Can you work these out from the model? Positions are in its coordinate system, mm. Face numbers are marked on the shaded views. A direction names the side the tool comes from. Coordinates: 2 decimals unless noted, no trailing zeros.
```python
from build123d import *

# Parameters (mm, degrees)
SKETCH1_R                    = 9.5
BOSS_EXTRUDE1_DEPTH          = 10
CHAMFER1_SIZE                = 0.75
CIRPATTERN1_COUNT            = 12
CHAMFER1_OF_CIRPATTERN1_SIZE = 0.75
SKETCH2_R                    = 7
SKETCH2_R_2                  = 4.5
CUT_EXTRUDE1_DEPTH           = 2
FILLET1_R                    = 1
FILLET1_OF_MIRROR1_R         = 1
CUT_EXTRUDE2_REACH           = 24.181


with BuildPart() as part:
    # Sketch1 → Boss-Extrude1 (new body)
    with BuildSketch(Plane.XY):
        Circle(SKETCH1_R)
        with BuildLine():
            ThreePointArc((-2.07, 9.271736623), (0, 9.5), (2.07, 9.271736623))
            ThreePointArc((2.07, 9.271736623), (1.625653209, 11.72726856), (0.57, 13.988391616))
            ThreePointArc((0.57, 13.988391616), (0, 14), (-0.57, 13.988391616))
            ThreePointArc((-0.57, 13.988391616), (-1.625653209, 11.72726856), (-2.07, 9.271736623))
        make_face()
    boss_extrude1 = extrude(amount=BOSS_EXTRUDE1_DEPTH)

    # Chamfer1
    chamfer1_edges = [part.edges().sort_by_distance(p)[0] for p in [
        (0, 14, 10),
        (0, 14, 0),
    ]]
    chamfer(chamfer1_edges, length=CHAMFER1_SIZE)

    # CirPattern1: Boss-Extrude1 ×12 about axis
    cirpattern1_axis = Axis((0, 0, 0), (0, 0, 1))
    for i in range(1, CIRPATTERN1_COUNT):
        add(boss_extrude1.rotate(cirpattern1_axis, i * 360 / CIRPATTERN1_COUNT))

    # Chamfer1 of CirPattern1
    chamfer1_of_cirpattern1_edges = [part.edges().sort_by_distance(p)[0] for p in [
        (-7, 12.124355653, 10),
        (-7, 12.124355653, 0),
        (-12.124355653, 7, 10),
        (-12.124355653, 7, 0),
        (-14, 0, 10),
        (-14, 0, 0),
        (-12.124355653, -7, 10),
        (-12.124355653, -7, 0),
        (-7, -12.124355653, 10),
        (-7, -12.124355653, 0),
        (0, -14, 10),
        (0, -14, 0),
        (7, -12.124355653, 10),
        (7, -12.124355653, 0),
        (12.124355653, -7, 10),
        (12.124355653, -7, 0),
        (14, 0, 10),
        (14, 0, 0),
        (12.124355653, 7, 10),
        (12.124355653, 7, 0),
        (7, 12.124355653, 10),
        (7, 12.124355653, 0),
    ]]
    chamfer(chamfer1_of_cirpattern1_edges, length=CHAMFER1_OF_CIRPATTERN1_SIZE)

    # Sketch2 → Cut-Extrude1 (cut)
    with BuildSketch(Plane.XY.offset(10)):
        Circle(SKETCH2_R)
        Circle(SKETCH2_R_2, mode=Mode.SUBTRACT)
    cut_extrude1 = extrude(amount=-CUT_EXTRUDE1_DEPTH, mode=Mode.SUBTRACT)

    # Fillet1
    fillet1_edges = [part.edges().sort_by_distance(p)[0] for p in [
        (-7, 0, 8),
        (-4.5, 0, 8),
    ]]
    fillet(fillet1_edges, radius=FILLET1_R)

    # Mirror1: Cut-Extrude1 across plane
    add(cut_extrude1.mirror(Plane.XY.offset(5)), mode=Mode.SUBTRACT)

    # Fillet1 of Mirror1
    fillet1_of_mirror1_edges = [part.edges().sort_by_distance(p)[0] for p in [
        (-7, 0, 2),
        (-4.5, 0, 2),
    ]]
    fillet(fillet1_of_mirror1_edges, radius=FILLET1_OF_MIRROR1_R)

    # Sketch3 → Cut-Extrude2 (cut, up to next)
    with BuildSketch(Plane.XY.offset(10), mode=Mode.PRIVATE) as cut_extrude2_sk1:
        with BuildLine():
            Line((1.118033989, 1), (-1.118033989, 1))
            ThreePointArc((-1.118033989, 1), (-0.535233135, -1.401258538), (1.5, 0))
            ThreePointArc((1.5, 0), (1.401258538, 0.535233135), (1.118033989, 1))
        make_face()
    cut_extrude2_tool1 = extrude(cut_extrude2_sk1.sketch, amount=-CUT_EXTRUDE2_REACH, mode=Mode.PRIVATE) & part.part
    add(cut_extrude2_tool1.solids().sort_by_distance((0, -0.148024, 10))[0], mode=Mode.SUBTRACT)


solid = part.part
```
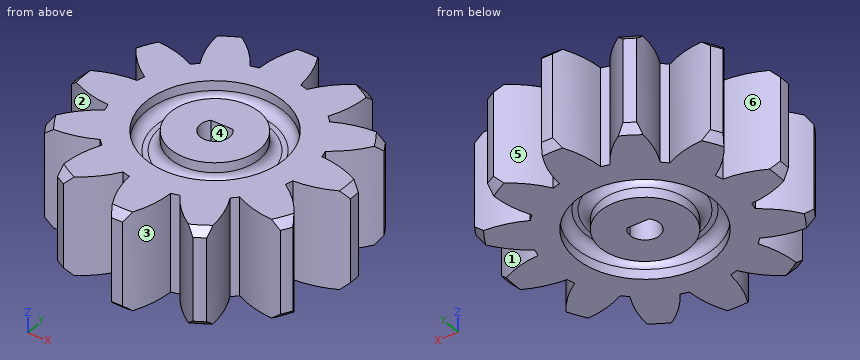
1. We'd pull the mould along X, two halves only. Please class the marked faces 1, 2 and 3: released by +X, released by -X, zero draft, split by the parting line, or undercut.
2. Which directions (+Z, -Z, +X, -X, +Y, -Y) give clear straight access to the entire face, cutting with the end or side of a thin tool? Please do the marked faces 4, 5 and 6.
3. I'm going to push flat-ended pins straight in: P1, Ø1.5, axis at y = 3.5, z = 3.5, coming from the +X side; P2, Ø4, axis at y = -10.5, z = 6.5, coming from the -X side; P3, Ø11, axis at x = 0, y = 0, coming from the +Z side; P4, Ø3, axis at x = 7.5, z = 5, coming from the -Y side. Where does each tip first touch, or does it pass through?
4. If I drill on L1, parallel to Y at x = 0, z = 9.25; L2, parallel to Y at x = 0, z = 0.25; L3, parallel to X at y = 11.25, z = 8.25, over which ranges is the centre line in solid material (lowest first)?
5. If we section it at A-A, the plane z = 1.5: Count the separate pieces of the cut face and the enclosed holes in it, plus the area to 3 significant figures.
Answers:
1. face 1: released by +X
1. face 2: released by -X
1. face 3: undercut
2. face 4: +Z, -Z
2. face 5: +Z, -Z, +Y
2. face 6: +Z, -Z, -X
3. P1: stops at x = 10.78
3. P2: stops at x = -7.5
3. P3: stops at z = 10
3. P4: stops at y = -12.4
4. L1: y = -14 to -7, -4.5 to -1.5, 1 to 4.5, 7 to 14
4. L2: y = -13.5 to -7, -4.5 to -1.5, 1 to 4.5, 7 to 13.5
4. L3: x = -7.49 to -4.78, -1.76 to 1.76, 4.78 to 7.49
5. separate pieces: 2
5. enclosed holes: 2
5. area: 364 mm2
